Autodesk Inventor part; units mm, degrees
ref_plane "YZ Plane" through (0, 0, 0) normal (1, 0, 0) x (0, 1, 0)
ref_plane "XZ Plane" through (0, 0, 0) normal (0, 1, 0) x (-1, 0, 0)
ref_plane "XY Plane" through (0, 0, 0) normal (0, 0, 1) x (1, 0, 0)
sketch "스케치1" plane through (0, 0, 0) normal (0, 1, 0) x (-1, 0, 0)
  circle A0 centre (0, 0) radius 2.5
  circle A1 centre (0, 0) radius 12.5
  circle A2 centre (0, 0) radius 10
  circle A3 centre (0, 0) radius 5
  dimension "d0" = 5
  dimension "d1" = 25
  dimension "d2" = 20
  dimension "d3" = 10
extrude "돌출1" add sketch "스케치1" along normal blind 2.5
sketch "스케치2" plane through (0, 2.5, 0) normal (0, 1, 0) x (1, 0, 0)
  line L0 (1, -11) -> (-1, -11)
  line L1 (-1, -11) -> (-1, 11)
  line L2 (-1, 11) -> (1, 11)
  line L3 (1, 11) -> (1, -11)
  circle A0 centre (0, 0) radius 10
  dimension "d6" = 1
  dimension "d7" = 1
  dimension "d8" = 1
  dimension "d9" = 1
extrude "돌출2" add sketch "스케치2" against normal blind 2.5 contours L0 L1 A0 L3 | A0 L1 L3 | A0 L1 L2 L3
pattern_circular "원형 패턴1" count 6 over 360 about axis through (0, 0, 0) along (0, 1, 0) of "돌출2"
sketch "스케치3" plane through (0, 2.5, 0) normal (0, 1, 0) x (1, 0, 0)
  line L0 (-2, 0) -> (-2.4843, 0.2796)
  circle A0 centre (0, 0) radius 2.5
extrude "돌출3" cut sketch "스케치3" against normal blind 2.5
fillet "모깎기1" radius 1 2 edges at (12.5, 2.5, 0) (12.5, 0, 0)
properties part number "보조바퀴"
CAD build for the part. Positions are in the model's coordinates, mm. Coordinates: 2 decimals unless noted, no trailing zeros. Write each loop counter-clockwise with the first axis right and the second up, starting at its lowest first coordinate (ties: lowest second). Pieces come first, ordered by that corner, then holes. Notation, with made-up numbers: M 11.5,5 L 26.5,5 A28 cw 26.5,39 Z; hole C 46.25,45.5 d1. An arc over 180 degrees is marked long. Answer as a JSON object with one key per item and string values. Group by question number.
1) Mould opens along X. For faces 1 (the face through (-5.96, 1.268, -4.596)), 2 (the face through (-11.923, 1.246, -3.755)) say: +X half, -X half, draft (parallel to the pull), parting line (faces both ways), or undercut.
2) Saw through at A-A (x = 0). Write the cut outline in (y, z).
3) Wall check: line 1 (Z direction, x = 7.25, y = 1.4); line 2 (X direction, y = 1.15, z = -3.25); line 3 (Z direction, x = 0, y = 1.2). Give the ranges that are in metal, low to high. Write a range as from..to.
4) Pin check, flat tips, straight feed: pin 1 Ø4 at (x, z) = (0, 0) entering from -Y; pin 2 Ø0.8 at (y, z) = (1, -7.5) entering from +X; pin 3 Ø0.8 at (y, z) = (1, -7.5) entering from -X; pin 4 Ø1.5 at (x, y) = (-2.5, 2) entering from +Z. Stop position of each tip, or through.
5) Saw through at C-C (y = 0.7). Write the cut outline in (x, z), plus the area to 3 significant figures.
6) Saw through at D-D (x = -7.25). Give the number of separate pieces and of enclosed holes in the cut face, plus the area to 3 significant figures.
7) Saw through at B-B (z = 0). Write the cut outline in (x, y).
Values follow:
{
 "1": {"face 1": "undercut", "face 2": "parting line"},
 "2": {"outline": "M 0,-11.5 A1 ccw 1,-12.5 L 1.5,-12.5 A1 ccw 2.5,-11.5 L 2.5,-2.5 L 0,-2.5 Z; M 0,2.5 L 2.5,2.5 L 2.5,11.5 A1 ccw 1.5,12.5 L 1,12.5 A1 ccw 0,11.5 Z"},
 "3": {"line 1": "z = -10.18..-6.89, -5.34..-3.03, 3.03..5.34, 6.89..10.18", "line 2": "x = -12.07..-9.46, -7.63..7.63, 9.46..12.07", "line 3": "z = -12.5..-2.5, 2.5..12.5"},
 "4": {"pin 1": "passes through", "pin 2": "stops at x = 10.29", "pin 3": "stops at x = -10.29", "pin 4": "stops at z = 12.35"},
 "5": {"outline": "C 0,0 d24.91; hole M -9.12,-4.11 L -4.74,-1.58 A5 cw -4.74,1.58 L -9.12,4.11 A10 ccw Z; hole M -8.12,-5.84 A10 ccw -1,-9.95 L -1,-4.9 A5 cw -3.74,-3.32 Z; hole M -8.12,5.84 L -3.74,3.32 A5 cw -1,4.9 L -1,9.95 A10 ccw Z; hole C 0,0 d5; hole M 1,-9.95 A10 ccw 8.12,-5.84 L 3.74,-3.32 A5 cw 1,-4.9 Z; hole M 1,4.9 A5 cw 3.74,3.32 L 8.12,5.84 A10 ccw 1,9.95 Z; hole M 4.74,-1.58 L 9.12,-4.11 A10 ccw 9.12,4.11 L 4.74,1.58 A5 cw Z", "area": "292 mm2"},
 "6": {"separate pieces": "4", "enclosed holes": "0", "area": "27.0 mm2"},
 "7": {"outline": "M -12.5,1 A1 ccw -11.5,0 L -10,0 L -10,2.5 L -11.5,2.5 A1 ccw -12.5,1.5 Z; M -5,0 L -2.5,0 L -2.5,2.5 L -5,2.5 Z; M 2.5,0 L 5,0 L 5,2.5 L 2.5,2.5 Z; M 10,0 L 11.5,0 A1 ccw 12.5,1 L 12.5,1.5 A1 ccw 11.5,2.5 L 10,2.5 Z"}
}
